from build123d import *

# Parameters (mm, degrees)
SKETCH2_W                    = 12.7
SKETCH2_H                    = 1.8034
SKETCH2_W_2                  = 8.0391
SKETCH2_H_2                  = 4.1783
SKETCH2_W_3                  = 15.0876
SKETCH2_H_3                  = 5.588
SKETCH2_R                    = 2.96545
BOSS_EXTRUDE1_DEPTH          = 3.048
SKETCH3_W                    = 12.7
SKETCH3_H                    = 0.2286
MADE_HOOD_SLOT_SMALLER_DEPTH = 3.048
SKETCH5_W                    = 3.0734
SKETCH5_H                    = 7.2898
CUT_EXTRUDE1_DEPTH           = 4.048
SKETCH7_W                    = 1.27
SKETCH7_H                    = 2.413
BOSS_EXTRUDE2_DEPTH          = 3.048


with BuildPart() as part:
    # Sketch2 → Boss-Extrude1 (new body)
    with BuildSketch(Plane(origin=(0, 0, 0), x_dir=(0, 0, -1), z_dir=(1, 0, 0))):
        Polygon((6.35, 24.0284), (0, 24.0284), (0, 21.1836), (-3.048, 21.1836), (-3.048, 16.1036), (0, 16.1036), (0, 9.8044), (-3.048, 9.8044), (-3.048, 4.7244), (6.35, 4.7244), (6.35, 1.5494), (46.863, 1.5494), (46.863, 4.7244), (84.963, 4.7244), (84.963, 12.0142), (86.7664, 12.0142), (86.7664, 4.7244), (89.3064, 4.7244), (89.3064, 27.2034), (64.77, 27.2034), (64.77, 24.0284), (53.213, 24.0284), (53.213, 27.2034), (6.35, 27.2034), align=None)
        with Locations((78.613, 23.6601)):
            Rectangle(SKETCH2_W, SKETCH2_H, mode=Mode.SUBTRACT)
        with Locations((10.64895, 7.29615)):
            Rectangle(SKETCH2_W_2, SKETCH2_H_2, mode=Mode.SUBTRACT)
        with Locations((31.8008, 9.7155)):
            Rectangle(SKETCH2_W_3, SKETCH2_H_3, mode=Mode.SUBTRACT)
        with Locations((53.48605, 9.17575)):
            Circle(SKETCH2_R, mode=Mode.SUBTRACT)
    extrude(amount=BOSS_EXTRUDE1_DEPTH)

    # Sketch3 → made hood slot smaller (add)
    with BuildSketch(Plane.ZY):
        with Locations((-78.613, 24.4475)):
            Rectangle(SKETCH3_W, SKETCH3_H)
    extrude(amount=-MADE_HOOD_SLOT_SMALLER_DEPTH)

    # Sketch5 → Cut-Extrude1 (cut, through all)
    with BuildSketch(Plane(origin=(3.048, 0, 0), x_dir=(0, 0, -1), z_dir=(1, 0, 0))):
        with Locations((86.4997, 8.3693)):
            Rectangle(SKETCH5_W, SKETCH5_H)
    extrude(amount=-CUT_EXTRUDE1_DEPTH, mode=Mode.SUBTRACT)

    # Sketch7 → Boss-Extrude2 (add)
    with BuildSketch(Plane(origin=(3.048, 0, 0), x_dir=(0, 0, -1), z_dir=(1, 0, 0))):
        Polygon((-3.048, 4.7244), (-3.048, 2.3114), (6.35, 2.3114), (6.35, -3.2766), (78.613, -3.2766), (78.613, 2.3114), (84.963, 2.3114), (84.963, 4.7244), align=None)
        with Locations((88.6714, 3.5179)):
            Rectangle(SKETCH7_W, SKETCH7_H)
    extrude(amount=-BOSS_EXTRUDE2_DEPTH)


solid = part.part
The model under review builds one solid part; all positions refer to its coordinate system, in mm. A direction names the side the tool comes from. Round coordinates to 2 decimals unless told otherwise and drop trailing zeros. Order: outer loops, then holes, each group sorted by start corner. A loop starts at its lowest first (then second) coordinate and runs counter-clockwise, first axis right, second up. Notation, with made-up numbers: (-2, -18.75) -> (15, -18.75) arc R31 ccw to (15, 19.25) -> close; hole circle Ø7 at (3, 69.5). An arc over 180 degrees is marked (long way). Write item = value, one per line. Start each with the question number.
Item 1: Consider section A-A on z = -82. Write out the cut boundary in (x, y).
Item 2: For faces 5 (the face through (2, 9.804, 2)), 6 (the face through (2, 26, -6.35)), 7 (the face through (2, 2.311, -2)), 8 (the face through (2, 22.758, -79)), list the 3-axis set-ups (+Z, -Z, +X, -X, +Y, -Y) from which the entire face can be reached by the end or side of a thin tool; tool diameter is ignored.
Item 3: Clearance check with flat-ended pins moving along their axes: pin 1 Ø0.9 at (x, z) = (1.5, -80.5) entering from -Y; pin 2 Ø3.5 at (y, z) = (9.18, -53.49) entering from +X; pin 3 Ø0.9 at (x, y) = (1, 25.5) entering from +Z. State where each tip first meets the part, or that it passes through.
Item 4: Consider section C-C on x = 1.8. Count the separate pieces of the cut face and the enclosed holes in it, plus the area to 3 significant figures.
Item 5: Consider section B-B on y = 3.5. Write out the cut boundary in (x, z).
Item 6: For line 1 along Z through (x, y) = (2.75, 9); line 2 along Y through (x, z) = (1.35, -75); line 3 along Y through (x, z) = (2.15, -81), list the stretches that pass through material, from the lowest coordinate up.
Item 7: Consider section D-D on z = -62.5. Write out the cut boundary in (x, y).
Item 8: Mouldability with a two-part tool opening along Z and no side actions: class faces 1 (the face through (2, 15, -89.306)), 2 (the face through (0, 12, -42)), 3 (the face through (2, 13, 0)), 4 (the face through (2, 24, -84.963)) as released by +Z, released by -Z, zero draft, split by the parting line, or undercut.
Conclusion:
q1.outline = (0, 2.31) -> (3.05, 2.31) -> (3.05, 22.76) -> (0, 22.76) -> close; (0, 24.33) -> (3.05, 24.33) -> (3.05, 27.2) -> (0, 27.2) -> close
q2.face_5 = +Z, +X, -X
q2.face_6 = +Z, +X, -X, +Y
q2.face_7 = +Z, +X, -X, -Y
q2.face_8 = +X, -X
q3.pin_1 = 2.31
q3.pin_2 = through
q3.pin_3 = -6.35
q4.separate_pieces = 1
q4.enclosed_holes = 4
q4.area = 2,410 mm2
q5.outline = (0, -89.31) -> (3.05, -89.31) -> (3.05, -88.04) -> (0, -88.04) -> close; (0, -84.96) -> (3.05, -84.96) -> (3.05, 3.05) -> (0, 3.05) -> close
q6.line_1 = -89.31 to -88.04, -84.96 to -56.45, -50.53 to -39.34, -24.26 to -14.67, -6.63 to 3.05
q6.line_2 = -3.28 to 22.76, 24.33 to 27.2
q6.line_3 = 2.31 to 22.76, 24.33 to 27.2
q7.outline = (0, -3.28) -> (3.05, -3.28) -> (3.05, 24.03) -> (0, 24.03) -> close
q8.face_1 = released by -Z
q8.face_2 = zero draft
q8.face_3 = released by +Z
q8.face_4 = undercut
